For this review, take the finished solid that the model builds, in its own axes (mm). Face numbers are marked on the shaded views. A direction names the side the tool comes from. Round coordinates to 2 decimals unless told otherwise and drop trailing zeros. Order: outer loops, then holes, each group sorted by start corner. A loop starts at its lowest first (then second) coordinate and runs counter-clockwise, first axis right, second up. Notation, with made-up numbers: (0.25, 47) - (11.25, 47) arc R8 ccw to (11.25, 52) - close; hole circle Ø9 at (82, 14). An arc over 180 degrees is marked (long way). One line per question, with ' | ' between items.
```python
from build123d import *

# Parameters (mm, degrees)
SKETCH3_W          = 31.75
SKETCH3_H          = 31.75
SKETCH3_W_2        = 12.7
SKETCH3_H_2        = 15.875
CUT_EXTRUDE1_DEPTH = 8.509


with BuildPart() as part:
    # Sketch1 → Revolve1 (revolve)
    with BuildSketch(Plane.XY):
        Polygon((-9.525, 0), (-9.525, 7.9375), (71.4248, 7.9375), (71.4248, 25.52065), (112.3442, 25.52065), (112.3442, 0), align=None)
    revolve(axis=Axis((112.3442, 0, 0), (-1, 0, 0)))

    # Sketch2 → Revolve2 (revolve)
    with BuildSketch(Plane.XY):
        with BuildLine():
            Line((-31.75, 0), (-31.75, 5.59435))
            Line((-31.75, 5.59435), (-30.99435, 6.35))
            Line((-30.99435, 6.35), (-13.2334, 6.35))
            Line((-13.2334, 6.35), (-12.726366704, 5.842966704))
            ThreePointArc((-12.726366704, 5.842966704), (-12.190743755, 5.485074892), (-11.558933409, 5.3594))
            Line((-11.558933409, 5.3594), (-11.176, 5.3594))
            ThreePointArc((-11.176, 5.3594), (-10.008566704, 5.842966704), (-9.525, 7.0104))
            Line((-9.525, 7.0104), (-9.525, 0))
            Line((-9.525, 0), (-31.75, 0))
        make_face()
    revolve(axis=Axis((-9.525, 0, 0), (-1, 0, 0)))

    # Sketch3 → Cut-Extrude1 (cut)
    with BuildSketch(Plane(origin=(-10.16, 0, 0), x_dir=(0, 0, -1), z_dir=(1, 0, 0))):
        Rectangle(SKETCH3_W, SKETCH3_H)
        Rectangle(SKETCH3_W_2, SKETCH3_H_2, mode=Mode.SUBTRACT)
    extrude(amount=CUT_EXTRUDE1_DEPTH, mode=Mode.SUBTRACT)


solid = part.part
```
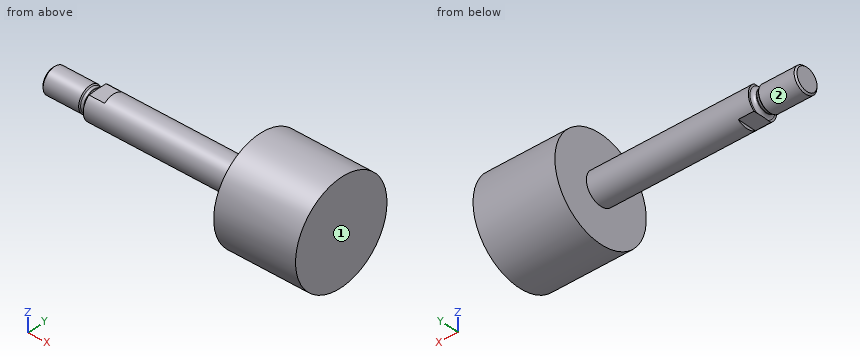
(1) Insertion check: pin 1 (1.3 mm diameter, centred on y = 0, z = -7.5, fed in from -X); pin 2 (3 mm diameter, centred on y = 7.5, z = 4.5, fed in from -X) (3 decimals); pin 3 (9 mm diameter, centred on x = -7, y = -2, fed in from +Z). Each pin has a flat end and moves straight along its axis. Give the tip position at first contact, or say it passes through.
Output values:
pin 1: x = -1.65 | pin 2: x = -9.525 | pin 3: z = 6.35
(2) We need section C-C on x = 13.5. State the section outline as (y, z) points (1 decimal), plus the area to 3 significant figures.
Output values:
outline: circle Ø15.9 at (0, 0) | area: 198 mm^2
(3) We need section D-D on z = 15. State the section outline as (x, y) points.
Output values:
outline: (71.42, -20.65) - (112.34, -20.65) - (112.34, 20.65) - (71.42, 20.65) - close
(4) For the marked faces 1 and 2, list the 3-axis set-ups (+Z, -Z, +X, -X, +Y, -Y) from which the entire face can be reached by the end or side of a thin tool; tool diameter is ignored.
Output values:
face 1: +Z, -Z, +X, +Y, -Y | face 2: -X
(5) We need section B-B on y = 0. State the section outline as (x, z) points.
Output values:
outline: (-31.75, -5.59) - (-30.99, -6.35) - (-13.23, -6.35) - (-12.73, -5.84) arc R1.65 cw to (-11.56, -5.36) - (-11.18, -5.36) arc R1.65 cw to (-9.66, -6.35) - (-1.65, -6.35) - (-1.65, -7.94) - (71.42, -7.94) - (71.42, -25.52) - (112.34, -25.52) - (112.34, 25.52) - (71.42, 25.52) - (71.42, 7.94) - (-1.65, 7.94) - (-1.65, 6.35) - (-9.66, 6.35) arc R1.65 cw to (-11.18, 5.36) - (-11.56, 5.36) arc R1.65 cw to (-12.73, 5.84) - (-13.23, 6.35) - (-30.99, 6.35) - (-31.75, 5.59) - close
(6) For probe 1 along X at (y, z) = (-10.5, -22.5); probe 2 along Z at (x, y) = (35.5, 0); probe 3 along Y at (x, z) = (65, -6), list the stretches that pass through material, from the lowest coordinate up. Write a range as [from, to].
Output values:
probe 1: [71.42, 112.34] | probe 2: [-7.94, 7.94] | probe 3: [-5.2, 5.2]
